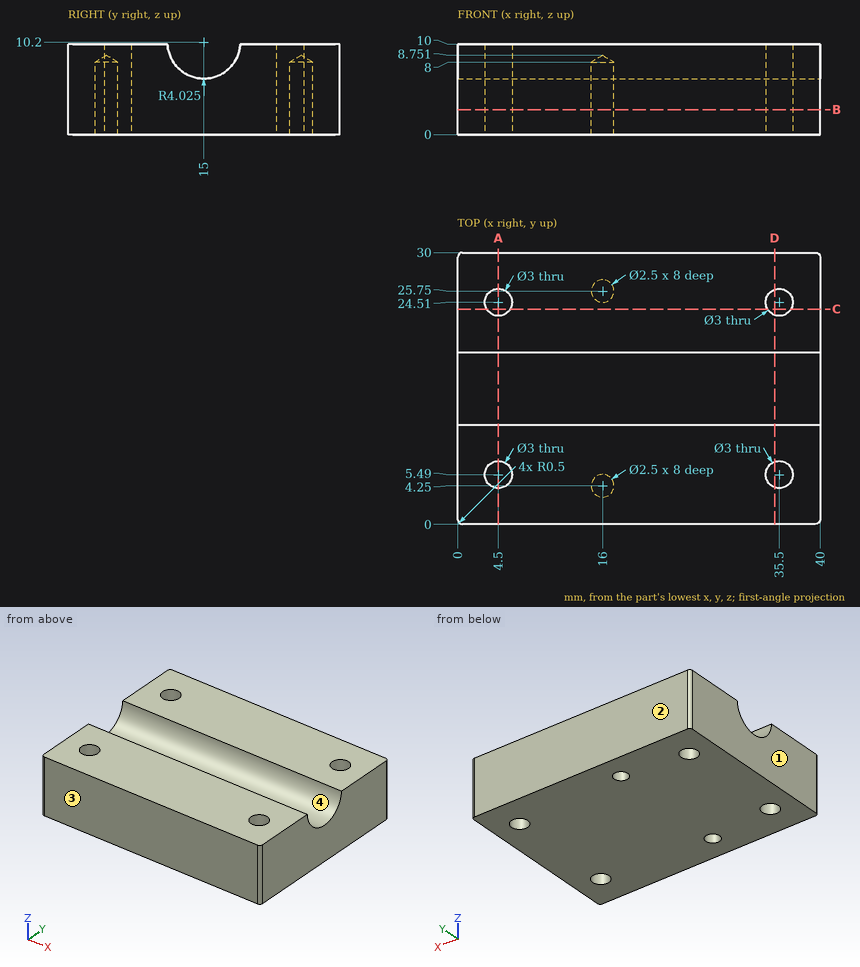
Geometry check sheet. Reference: drawing and pictorial views, mm from the part's lowest x, y, z. Give positions to 0.01 mm unless a question says otherwise; leave off trailing zeros. Write each loop counter-clockwise with the first axis right and the second up, starting at its lowest first coordinate (ties: lowest second). Pieces come first, ordered by that corner, then holes. Notation, with made-up numbers: M -16.75,-17.75 L 27.25,-17.75 A34 cw 27.25,14.25 Z; hole C -3,1 d7. An arc over 180 degrees is marked long. Put each result on its own line as item: value. Start each with the question number.
1. Scan lines: line 1 along Y through (x, z) = (4.5, 5.75); line 2 along Y through (x, z) = (16, 4.5); line 3 along X through (y, z) = (25.75, 3.5). Record each from-to range of solid material in increasing order. Write a range as [from, to].
2. Section check C-C (y = 23.75). Record the cut outline in (x, z), and give its area (3 significant figures).
3. Section check D-D (x = 35). Record the cut outline in (y, z) (3 decimals).
4. Section check A-A (x = 4.5). Record the cut outline in (y, z) (3 decimals).
5. Go/stop test with a flat-tipped pin: pin 1 Ø2.5 at (x, y) = (35.5, 24.51) entering from +Z. Record where the tip stops, or that it passes through.
6. Section check B-B (z = 2.75). Record the cut outline in (x, y), and give its area (3 significant figures).
7. Draft check along Y on the marked faces 1, 2, 3 and 4. Enter one of: +Y half, -Y half, draft (parallel to the pull), parting line (faces both ways), or undercut.
Answer list:
1. line 1: [0, 3.99], [6.99, 23.01], [26.01, 30]
1. line 2: [0, 3], [5.5, 24.5], [27, 30]
1. line 3: [0, 3.66], [5.34, 14.75], [17.25, 34.66], [36.34, 40]
2. outline: M 0,0 L 3.21,0 L 3.21,10 L 0,10 Z; M 5.79,0 L 34.21,0 L 34.21,10 L 5.79,10 Z; M 36.79,0 L 40,0 L 40,10 L 36.79,10 Z
2. area: 348 mm2
3. outline: M 0,0 L 4.076,0 L 4.076,10 L 0,10 Z; M 6.904,0 L 23.096,0 L 23.096,10 L 19.02,10 A4.025 cw 10.98,10 L 6.904,10 Z; M 25.924,0 L 30,0 L 30,10 L 25.924,10 Z
4. outline: M 0,0 L 3.99,0 L 3.99,10 L 0,10 Z; M 6.99,0 L 23.01,0 L 23.01,10 L 19.02,10 A4.025 cw 10.98,10 L 6.99,10 Z; M 26.01,0 L 30,0 L 30,10 L 26.01,10 Z
5. pin 1: through
6. outline: M 0,0.5 A0.5 ccw 0.5,0 L 39.5,0 A0.5 ccw 40,0.5 L 40,29.5 A0.5 ccw 39.5,30 L 0.5,30 A0.5 ccw 0,29.5 Z; hole C 4.5,5.49 d3; hole C 4.5,24.51 d3; hole C 16,4.25 d2.5; hole C 16,25.75 d2.5; hole C 35.5,5.49 d3; hole C 35.5,24.51 d3
6. area: 1,160 mm2
7. face 1: draft
7. face 2: +Y half
7. face 3: -Y half
7. face 4: undercut
